from build123d import *

# Parameters (mm, degrees)
F0_W      = 53.975
F0_H      = 12.7
F1_DEPTH  = 3.175
F3_DEPTH  = 9.525
F4_R      = 3.175
F5_DEPTH  = 3.176
F6_W      = 53.975
F6_H      = 19.05
F7_DEPTH  = 25.4
F8_W      = 53.975
F8_H      = 31.75
F9_DEPTH  = 3.175
F11_DEPTH = 25.401
F12_R     = 3.175
F13_DEPTH = 9.525
F15_DEPTH = 15.4432


# Not quite as in the source:
# - a length typed as a fraction of an inch, garbled in the dataset ("3 / 203.2 mm" for 3/8 in), is restored


with BuildPart() as f1:
    # F0 (on Front) → F1 (new body)
    with BuildSketch(Plane.XZ):
        with Locations((-7.6144175836, -40.016034618)):
            Rectangle(F0_W, F0_H)
    extrude(amount=F1_DEPTH)

    # F2 (on face) → F3 (join)
    with BuildSketch(Plane.XZ.offset(3.175)):
        with BuildLine():
            ThreePointArc((-25.0769175836, -40.016034618), (-28.2519175836, -36.841034618), (-31.4269175836, -40.016034618))
            ThreePointArc((-31.4269175836, -40.016034618), (-28.2519175836, -43.191034618), (-25.0769175836, -40.016034618))
        make_face()
    extrude(amount=F3_DEPTH)

    # F4 (on face) → F5 (cut, through all)
    with BuildSketch(Plane.XZ.offset(3.175)):
        with Locations((13.0230824164, -40.016034618)):
            Circle(F4_R)
    extrude(amount=-F5_DEPTH, mode=Mode.SUBTRACT)

    # F6 (on face) → F7 (join)
    with BuildSketch(Plane.XZ.offset(3.175)):
        with Locations((-7.6144175836, -24.141034618)):
            Rectangle(F6_W, F6_H)
    extrude(amount=-F7_DEPTH)

    # F8 (on face) → F9 (join)
    with BuildSketch(Plane.XZ.offset(3.175)):
        with Locations((-7.6144175836, 1.258965382)):
            Rectangle(F8_W, F8_H)
    extrude(amount=-F9_DEPTH)

    # F10 (on face) → F11 (cut, through all)
    with BuildSketch(Plane.XZ.offset(3.175)):
        with BuildLine():
            ThreePointArc((-25.0769175836, 10.783965382), (-28.2519175836, 13.958965382), (-31.4269175836, 10.783965382))
            ThreePointArc((-31.4269175836, 10.783965382), (-28.2519175836, 7.608965382), (-25.0769175836, 10.783965382))
        make_face()
    extrude(amount=-F11_DEPTH, mode=Mode.SUBTRACT)

    # F12 (on face) → F13 (join)
    with BuildSketch(Plane.XZ.offset(3.175)):
        with Locations((13.0230824164, 10.783965382)):
            Circle(F12_R)
    extrude(amount=F13_DEPTH)

    # F14 (on face) → F15 (cut)
    with BuildSketch(Plane(origin=(0, 0, 0), x_dir=(-1, 0, 0), z_dir=(0, 1, 0))):
        with BuildLine():
            ThreePointArc((-15.4106824164, 10.783965382), (-13.0230824164, 8.396365382), (-10.6354824164, 10.783965382))
            ThreePointArc((-10.6354824164, 10.783965382), (-13.0230824164, 13.171565382), (-15.4106824164, 10.783965382))
        make_face()
    extrude(amount=-F15_DEPTH, mode=Mode.SUBTRACT)


solid = f1.part
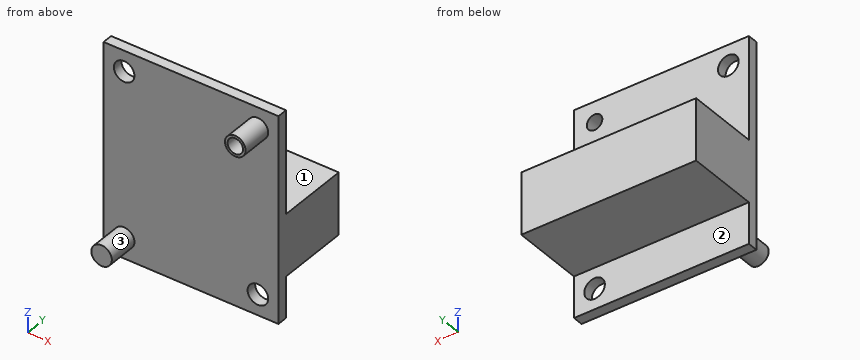
For this review, take the finished solid that the model builds, in its own axes (mm). Face numbers are marked on the shaded views. A direction names the side the tool comes from. Round coordinates to 2 decimals unless told otherwise and drop trailing zeros. Order: outer loops, then holes, each group sorted by start corner. A loop starts at its lowest first (then second) coordinate and runs counter-clockwise, first axis right, second up. Notation, with made-up numbers: (27.5, 77.5) -> (50.5, 77.5) arc R15 ccw to (50.5, 101.5) -> close; hole circle Ø1 at (22, 55.25). An arc over 180 degrees is marked (long way). Put each result on its own line as item: value.
Q1. For probe 1 along Y at (x, z) = (4, 1.5) (3 decimals); probe 2 along Z at (x, y) = (-6.5, 17.5); probe 3 along Y at (x, z) = (14, -32.5) (3 decimals), list the stretches that pass through material, from the lowest coordinate up. Write a range as [from, to].
Check result:
probe 1: [-3.175, 0]
probe 2: [-33.67, -14.62]
probe 3: [-3.175, 22.225]
Q2. Add section A-A on z = 10. Write out the cut boundary in (x, y) (3 decimals), plus the area to 3 significant figures.
Check result:
outline: (-34.602, -3.175) -> (-31.329, -3.175) -> (-31.329, 0) -> (-34.602, 0) -> close; (-25.175, -3.175) -> (9.946, -3.175) -> (9.946, -12.7) -> (10.768, -12.7) -> (10.768, 0) -> (-25.175, 0) -> close; (15.278, -12.7) -> (16.1, -12.7) -> (16.1, -3.175) -> (19.373, -3.175) -> (19.373, 0) -> (15.278, 0) -> close
area: 153 mm2
Q3. Add section B-B on x = -16. Write out the cut boundary in (y, z) (3 decimals), plus the area to 3 significant figures.
Check result:
outline: (-3.175, -46.366) -> (0, -46.366) -> (0, -33.666) -> (22.225, -33.666) -> (22.225, -14.616) -> (0, -14.616) -> (0, 17.134) -> (-3.175, 17.134) -> close
area: 625 mm2
Q4. Add section D-D on z = 3. Write out the cut boundary in (x, y) (3 decimals), plus the area to 3 significant figures.
Check result:
outline: (-34.602, -3.175) -> (19.373, -3.175) -> (19.373, 0) -> (-34.602, 0) -> close
area: 171 mm2
Q5. Insertion check: pin 1 Ø6 at (x, y) = (14, -8.5) entering from -Z; pin 2 Ø6.5 at (x, z) = (3.5, -43) entering from +Y; pin 3 Ø4 at (x, y) = (4.5, 5) entering from -Z. Each pin has a flat end and moves straight along its axis. Give the tip position at first contact, or say it passes through.
Check result:
pin 1: z = 7.61
pin 2: y = 0
pin 3: z = -33.67
Q6. Machinability: for the marked faces 1, 2 and 3, which of the approach directions +Z, -Z, +X, -X, +Y, -Y give a long, thin tool a straight path to every point of the face, cutting with its end or side? Answer none if there is none.
Check result:
face 1: +Z, +X, -X, +Y
face 2: -Z, +X, -X, +Y
face 3: -Y
Q7. Add section C-C on y = -1. Write out the cut boundary in (x, z) (3 decimals), plus the area to 3 significant figures.
Check result:
outline: (-34.602, -46.366) -> (19.373, -46.366) -> (19.373, 17.134) -> (-34.602, 17.134) -> close; hole circle Ø6.35 at (-28.252, 10.784); hole circle Ø6.35 at (13.023, -40.016); hole circle Ø4.775 at (13.023, 10.784)
area: 3,350 mm2
